```python
from build123d import *

# Parameters (mm, degrees)
BOSS_EXTRUDE1_DEPTH = 5
SKETCH2_R           = 8
BOSS_EXTRUDE2_DEPTH = 157
FILLET1_R           = 10
CUT_EXTRUDE1_DEPTH  = 30
SKETCH5_R           = 10
CUT_EXTRUDE2_DEPTH  = 1.5
FILLET2_SIZE        = 5
FILLET2_SIZE_2      = 1
FILLET4_R           = 1


with BuildPart() as part:
    # Sketch1 → Boss-Extrude1 (new, symmetric)
    with BuildSketch(Plane.XY):
        with BuildLine():
            Line((0, 78.5), (0, -78.5))
            Line((0, -78.5), (-21.9089023, -78.5))
            ThreePointArc((-21.9089023, -78.5), (-81.5, 0), (-21.9089023, 78.5))
            Line((-21.9089023, 78.5), (0, 78.5))
        make_face()
    extrude(amount=BOSS_EXTRUDE1_DEPTH, both=True)

    # Sketch2 → Boss-Extrude2 (add)
    with BuildSketch(Plane(origin=(0, 78.5, 0), x_dir=(1, 0, 0), z_dir=(0, 1, 0))):
        Circle(SKETCH2_R)
    extrude(amount=-BOSS_EXTRUDE2_DEPTH)

    # Fillet1
    fillet1_edges = [part.edges().sort_by_distance(p)[0] for p in [
        (-6.244997998, 0, -5),
        (-6.244997998, 0, 5),
    ]]
    fillet(fillet1_edges, radius=FILLET1_R)

    # Sketch3 → Cut-Extrude1 (cut)
    with BuildSketch(Plane.XZ.offset(78.5)):
        Polygon((2.5, -4.330127019), (5, 0), (2.5, 4.330127019), (-2.5, 4.330127019), (-5, 0), (-2.5, -4.330127019), align=None)
    cut_extrude1 = extrude(amount=-CUT_EXTRUDE1_DEPTH, mode=Mode.SUBTRACT)

    # Sketch5 → Cut-Extrude2 (cut)
    with BuildSketch(Plane.XZ.offset(78.5)):
        Circle(SKETCH5_R)
    cut_extrude2 = extrude(amount=-CUT_EXTRUDE2_DEPTH, mode=Mode.SUBTRACT)

    # Mirror1: Cut-Extrude1, Cut-Extrude2 across plane
    add(cut_extrude1.mirror(Plane.ZX), mode=Mode.SUBTRACT)
    add(cut_extrude2.mirror(Plane.ZX), mode=Mode.SUBTRACT)

    # Fillet2
    # an asymmetric fillet: 5, 1 mm, written as the material it takes off along each edge
    with BuildSketch(Plane(origin=(0, 0, 5), x_dir=(-0.11834786572698561, -0.9929721963266983, 0), z_dir=(0.9929721963266983, -0.11834786572698561, 0))) as fillet2_piece_1:
        with BuildLine():
            Bezier((81.5, FILLET2_SIZE), (81.5, 0), (81.5 - FILLET2_SIZE_2, 0), weights=[1, 0.707106781, 1])
            Line((81.5 - FILLET2_SIZE_2, 0), (81.5, 0))
            Line((81.5, 0), (81.5, FILLET2_SIZE))
        make_face()
    revolve(axis=Axis((0, 0, 5), (0, 0, -1)), revolution_arc=166.406474405, mode=Mode.SUBTRACT)
    with BuildSketch(Plane(origin=(0, 0, -5), x_dir=(-0.11834786572698561, -0.9929721963266983, 0), z_dir=(0.9929721963266983, -0.11834786572698561, 0))) as fillet2_piece_2:
        with BuildLine():
            Bezier((81.5 - FILLET2_SIZE_2, 0), (81.5, 0), (81.5, -FILLET2_SIZE), weights=[1, 0.707106781, 1])
            Line((81.5, -FILLET2_SIZE), (81.5, 0))
            Line((81.5, 0), (81.5 - FILLET2_SIZE_2, 0))
        make_face()
    revolve(axis=Axis((0, 0, -5), (0, 0, -1)), revolution_arc=166.406474405, mode=Mode.SUBTRACT)

    # Fillet4
    fillet4_edges = [part.edges().sort_by_distance(p)[0] for p in [
        (-3.75, 77, -2.165063509),
        (-10, 78.5, 0),
        (3.75, 77, -2.165063509),
        (0, 77, -4.330127019),
        (-3.75, 77, 2.165063509),
        (0, 77, 4.330127019),
        (3.75, 77, 2.165063509),
        (3.75, -77, -2.165063509),
        (-10, -78.5, 0),
        (0, -77, -4.330127019),
        (-3.75, -77, -2.165063509),
        (-3.75, -77, 2.165063509),
        (0, -77, 4.330127019),
        (3.75, -77, 2.165063509),
    ]]
    fillet(fillet4_edges, radius=FILLET4_R)


solid = part.part
```
Here's how the part is built. I have some questions about the finished solid (model axes, mm). A direction names the side the tool comes from. Give positions to 0.01 mm unless a question says otherwise; leave off trailing zeros. Write each loop counter-clockwise with the first axis right and the second up, starting at its lowest first coordinate (ties: lowest second). Pieces come first, ordered by that corner, then holes. Notation, with made-up numbers: M 76,17 L 91,17 A10 cw 91,27 Z; hole C 27,-40 d8. An arc over 180 degrees is marked long. Put each result on its own line as item: value. Start each with the question number.
Item 1: Will these pins go through, and if not, where does the flat tip stop? pin 1 (1 mm diameter, centred on x = -30.5, y = 17, fed in from -Z); pin 2 (5 mm diameter, centred on x = -1.5, z = 3.5, fed in from -Y); pin 3 (2.5 mm diameter, centred on x = 0.5, z = 2, fed in from +Y).
Item 2: Thinking about a two-plate mould opening in Z: for faces 4 (the flat face through (3.73, -62.44, -2.2)), 5 (the cylindrical face through (8, 1, 0)), 6 (the flat face through (-37, 1, 5)), which applies, +Z half, -Z half, draft (parallel to the pull), parting line (faces both ways), or undercut?
Item 3: If we section it at A-A, the plane x = 0: Write out the boundary of the cut face in (y, z), then the cut area to 3 significant figures.
Item 4: On a 3-axis mill with a long thin cutter (end or side, diameter ignored), from which of +Z, -Z, +X, -X, +Y, -Y can I reach the whole of each face in a straight line? I mean faces 1 (the flat face through (-3.77, 62.44, -2.13)), 2 (the flat face through (-3.73, -62.44, 2.2)), 3 (the flat face through (-16, 78.5, 0)). Say none if no direction works.
Item 5: I need wall thicknesses on L1, parallel to Z at x = -21, y = -66.5; L2, parallel to X at y = -24, z = -3.25; L3, parallel to X at y = 27, z = 3. Which ranges of each line are inside material? Lowest first, please. Write a range as from..to.
Item 6: If we section it at B-B, the plane x = -16: Write out the boundary of the cut face in (y, z), then the cut area to 3 significant figures.
Values:
1. pin 1: z = -5
1. pin 2: y = -77
1. pin 3: y = 48.5
2. face 4: undercut
2. face 5: parting line
2. face 6: +Z half
3. outline: M -77,-8 L 77,-8 L 77,-5.33 A1 ccw 76,-4.33 L 48.5,-4.33 L 48.5,4.33 L 76,4.33 A1 ccw 77,5.33 L 77,8 L -77,8 L -77,5.33 A1 ccw -76,4.33 L -48.5,4.33 L -48.5,-4.33 L -76,-4.33 A1 ccw -77,-5.33 Z
3. area: 1,970 mm²
4. face 1: +Y
4. face 2: -Y
4. face 3: +Z, -Z, +X, -X, +Y
5. L1: -5..5
5. L2: -77.63..7.31
5. L3: -76.69..7.42
6. outline: M -78.5,-5 L 78.5,-5 L 78.5,5 L -78.5,5 Z
6. area: 1,570 mm²
